Design review of the part built by this model. Coordinates are the model's own, in mm. Round coordinates to 2 decimals unless told otherwise and drop trailing zeros. Write each loop counter-clockwise with the first axis right and the second up, starting at its lowest first coordinate (ties: lowest second). Pieces come first, ordered by that corner, then holes.
from build123d import *

# Parameters (mm, degrees)
SKETCH1_R           = 68.58
SKETCH1_R_2         = 22.225
BOSS_EXTRUDE1_DEPTH = 3.175
SKETCH2_R           = 6.35
CUT_EXTRUDE1_DEPTH  = 3.175
CIRPATTERN1_COUNT   = 8


with BuildPart() as part:
    # Sketch1 → Boss-Extrude1 (new body)
    with BuildSketch(Plane(origin=(0, 0, 0), x_dir=(1, 0, 0), z_dir=(0, 1, 0))):
        Circle(SKETCH1_R)
        Circle(SKETCH1_R_2, mode=Mode.SUBTRACT)
    extrude(amount=BOSS_EXTRUDE1_DEPTH)

    # Sketch2 → Cut-Extrude1 (cut)
    with BuildSketch(Plane(origin=(0, 3.175, 0), x_dir=(1, 0, 0), z_dir=(0, 1, 0))):
        with Locations((0, 44.45)):
            Circle(SKETCH2_R)
    cut_extrude1 = extrude(amount=-CUT_EXTRUDE1_DEPTH, mode=Mode.SUBTRACT)

    # CirPattern1: Cut-Extrude1 ×8 about axis
    cirpattern1_axis = Axis((0, 0, 0), (0, 1, 0))
    for i in range(1, CIRPATTERN1_COUNT):
        add(cut_extrude1.rotate(cirpattern1_axis, i * 360 / CIRPATTERN1_COUNT), mode=Mode.SUBTRACT)


solid = part.part
1) Add section B-B on x = 0. State the section outline as (y, z) points (3 decimals).
2) For line 1 along X through (y, z) = (1.1, 0) (3 decimals); line 2 along X through (y, z) = (2.9, -34.5), list the stretches that pass through material, from the lowest coordinate up.
3) Add section D-D on y = 0.9. Count the separate pieces of the cut face and the enclosed holes in it, and give its area (3 significant figures).
4) The part is to be moulded in two halves that separate along Z. For faces 1 (the face through (36.868, 1.565, -57.827)), 2 (the face through (-16, 3.175, -16)), 3 (the face through (-36.467, 1.61, -35.298)), say which applies: pulls with the +Z half, pulls with the -Z half, needs draft (parallel to the pull), parting line crosses it, or undercut.
5) Add section C-C on x = 31.5. State the section outline as (y, z) points (3 decimals).
6) Add section A-A on z = 0. State the section outline as (x, y) points (3 decimals), and give its area (3 significant figures).
Computed:
1. outline: (0, -68.58) - (3.175, -68.58) - (3.175, -50.8) - (0, -50.8) - close; (0, -38.1) - (3.175, -38.1) - (3.175, -22.225) - (0, -22.225) - close; (0, 22.225) - (3.175, 22.225) - (3.175, 38.1) - (0, 38.1) - close; (0, 50.8) - (3.175, 50.8) - (3.175, 68.58) - (0, 68.58) - close
2. line 1: x = -68.58 to -50.8, -38.1 to -22.225, 22.225 to 38.1, 50.8 to 68.58
2. line 2: x = -59.27 to -36.99, -25.87 to 25.87, 36.99 to 59.27
3. separate pieces: 1
3. enclosed holes: 9
3. area: 12,200 mm2
4. face 1: parting line crosses it
4. face 2: needs draft
4. face 3: undercut
5. outline: (0, -60.918) - (3.175, -60.918) - (3.175, -37.781) - (0, -37.781) - close; (0, -25.081) - (3.175, -25.081) - (3.175, 25.081) - (0, 25.081) - close; (0, 37.781) - (3.175, 37.781) - (3.175, 60.918) - (0, 60.918) - close
6. outline: (-68.58, 0) - (-50.8, 0) - (-50.8, 3.175) - (-68.58, 3.175) - close; (-38.1, 0) - (-22.225, 0) - (-22.225, 3.175) - (-38.1, 3.175) - close; (22.225, 0) - (38.1, 0) - (38.1, 3.175) - (22.225, 3.175) - close; (50.8, 0) - (68.58, 0) - (68.58, 3.175) - (50.8, 3.175) - close
6. area: 214 mm2
